For this review, take the finished solid that the model builds, in its own axes (mm). Round coordinates to 2 decimals unless told otherwise and drop trailing zeros. Order: outer loops, then holes, each group sorted by start corner. A loop starts at its lowest first (then second) coordinate and runs counter-clockwise, first axis right, second up. Notation, with made-up numbers: (37.5, -23) -> (59.5, -23) arc R21 ccw to (59.5, 7) -> close; hole circle Ø6 at (87, 33.5). An arc over 180 degrees is marked (long way). Put each result on its own line as item: value. Start each with the question number.
```python
from build123d import *

# Parameters (mm, degrees)
F0_W     = 14
F0_H     = 14
F1_DEPTH = 2


with BuildPart() as f1:
    # F0 (on Front) → F1 (new body)
    with BuildSketch(Plane.XZ):
        with BuildLine():
            Line((154, 60.5), (-154, 60.5))
            ThreePointArc((-154, 60.5), (-157.535534, 59.035534), (-159, 55.5))
            Line((-159, 55.5), (-159, -55.5))
            ThreePointArc((-159, -55.5), (-157.535534, -59.035534), (-154, -60.5))
            Line((-154, -60.5), (154, -60.5))
            ThreePointArc((154, -60.5), (157.535534, -59.035534), (159, -55.5))
            Line((159, -55.5), (159, 55.5))
            ThreePointArc((159, 55.5), (157.535534, 59.035534), (154, 60.5))
        make_face()
        with Locations((-127, -28.5)):
            Rectangle(F0_W, F0_H, mode=Mode.SUBTRACT)
        with Locations((-108, -28.5)):
            Rectangle(F0_W, F0_H, mode=Mode.SUBTRACT)
        with Locations((-89, -28.5)):
            Rectangle(F0_W, F0_H, mode=Mode.SUBTRACT)
        with Locations((-127, -9.5)):
            Rectangle(F0_W, F0_H, mode=Mode.SUBTRACT)
        with Locations((-108, -9.5)):
            Rectangle(F0_W, F0_H, mode=Mode.SUBTRACT)
        with Locations((-89, -9.5)):
            Rectangle(F0_W, F0_H, mode=Mode.SUBTRACT)
        with Locations((-70, -28.5)):
            Rectangle(F0_W, F0_H, mode=Mode.SUBTRACT)
        with Locations((-51, -28.5)):
            Rectangle(F0_W, F0_H, mode=Mode.SUBTRACT)
        with Locations((-32, -28.5)):
            Rectangle(F0_W, F0_H, mode=Mode.SUBTRACT)
        with Locations((-70, -9.5)):
            Rectangle(F0_W, F0_H, mode=Mode.SUBTRACT)
        with Locations((-51, -9.5)):
            Rectangle(F0_W, F0_H, mode=Mode.SUBTRACT)
        with Locations((-32, -9.5)):
            Rectangle(F0_W, F0_H, mode=Mode.SUBTRACT)
        with Locations((32, -28.5)):
            Rectangle(F0_W, F0_H, mode=Mode.SUBTRACT)
        with Locations((51, -28.5)):
            Rectangle(F0_W, F0_H, mode=Mode.SUBTRACT)
        with Locations((70, -28.5)):
            Rectangle(F0_W, F0_H, mode=Mode.SUBTRACT)
        with Locations((32, -9.5)):
            Rectangle(F0_W, F0_H, mode=Mode.SUBTRACT)
        with Locations((51, -9.5)):
            Rectangle(F0_W, F0_H, mode=Mode.SUBTRACT)
        with Locations((70, -9.5)):
            Rectangle(F0_W, F0_H, mode=Mode.SUBTRACT)
        with Locations((89, -28.5)):
            Rectangle(F0_W, F0_H, mode=Mode.SUBTRACT)
        with Locations((108, -28.5)):
            Rectangle(F0_W, F0_H, mode=Mode.SUBTRACT)
        with Locations((127, -28.5)):
            Rectangle(F0_W, F0_H, mode=Mode.SUBTRACT)
        with Locations((89, -9.5)):
            Rectangle(F0_W, F0_H, mode=Mode.SUBTRACT)
        with Locations((108, -9.5)):
            Rectangle(F0_W, F0_H, mode=Mode.SUBTRACT)
        with Locations((127, -9.5)):
            Rectangle(F0_W, F0_H, mode=Mode.SUBTRACT)
        with Locations((-127, 9.5)):
            Rectangle(F0_W, F0_H, mode=Mode.SUBTRACT)
        with Locations((-108, 9.5)):
            Rectangle(F0_W, F0_H, mode=Mode.SUBTRACT)
        with Locations((-89, 9.5)):
            Rectangle(F0_W, F0_H, mode=Mode.SUBTRACT)
        with Locations((-127, 28.5)):
            Rectangle(F0_W, F0_H, mode=Mode.SUBTRACT)
        with Locations((-108, 28.5)):
            Rectangle(F0_W, F0_H, mode=Mode.SUBTRACT)
        with Locations((-89, 28.5)):
            Rectangle(F0_W, F0_H, mode=Mode.SUBTRACT)
        with Locations((-70, 9.5)):
            Rectangle(F0_W, F0_H, mode=Mode.SUBTRACT)
        with Locations((-51, 9.5)):
            Rectangle(F0_W, F0_H, mode=Mode.SUBTRACT)
        with Locations((-32, 9.5)):
            Rectangle(F0_W, F0_H, mode=Mode.SUBTRACT)
        with Locations((-70, 28.5)):
            Rectangle(F0_W, F0_H, mode=Mode.SUBTRACT)
        with Locations((-51, 28.5)):
            Rectangle(F0_W, F0_H, mode=Mode.SUBTRACT)
        with Locations((-32, 28.5)):
            Rectangle(F0_W, F0_H, mode=Mode.SUBTRACT)
        with Locations((32, 9.5)):
            Rectangle(F0_W, F0_H, mode=Mode.SUBTRACT)
        with Locations((51, 9.5)):
            Rectangle(F0_W, F0_H, mode=Mode.SUBTRACT)
        with Locations((70, 9.5)):
            Rectangle(F0_W, F0_H, mode=Mode.SUBTRACT)
        with Locations((32, 28.5)):
            Rectangle(F0_W, F0_H, mode=Mode.SUBTRACT)
        with Locations((51, 28.5)):
            Rectangle(F0_W, F0_H, mode=Mode.SUBTRACT)
        with Locations((70, 28.5)):
            Rectangle(F0_W, F0_H, mode=Mode.SUBTRACT)
        with Locations((89, 9.5)):
            Rectangle(F0_W, F0_H, mode=Mode.SUBTRACT)
        with Locations((108, 9.5)):
            Rectangle(F0_W, F0_H, mode=Mode.SUBTRACT)
        with Locations((127, 9.5)):
            Rectangle(F0_W, F0_H, mode=Mode.SUBTRACT)
        with Locations((89, 28.5)):
            Rectangle(F0_W, F0_H, mode=Mode.SUBTRACT)
        with Locations((108, 28.5)):
            Rectangle(F0_W, F0_H, mode=Mode.SUBTRACT)
        with Locations((127, 28.5)):
            Rectangle(F0_W, F0_H, mode=Mode.SUBTRACT)
    extrude(amount=F1_DEPTH)


solid = f1.part
```
Item 1: Consider section A-A, the plane x = -67. Write out the cut boundary in (y, z).
Item 2: Consider section B-B, the plane z = -12.5. Count the separate pieces of the cut face and the enclosed holes in it, plus the area to 3 significant figures.
Item 3: For L1, parallel to Z at x = 93, y = -1.45, list the stretches that pass through material, from the lowest coordinate up.
Evaluation:
1. outline: (-2, -60.5) -> (0, -60.5) -> (0, -35.5) -> (-2, -35.5) -> close; (-2, -21.5) -> (0, -21.5) -> (0, -16.5) -> (-2, -16.5) -> close; (-2, -2.5) -> (0, -2.5) -> (0, 2.5) -> (-2, 2.5) -> close; (-2, 16.5) -> (0, 16.5) -> (0, 21.5) -> (-2, 21.5) -> close; (-2, 35.5) -> (0, 35.5) -> (0, 60.5) -> (-2, 60.5) -> close
2. separate pieces: 13
2. enclosed holes: 0
2. area: 300 mm^2
3. L1: z = -60.5 to -35.5, -21.5 to -16.5, -2.5 to 2.5, 16.5 to 21.5, 35.5 to 60.5
